Here's the drawing with two shaded views (mm, measured from the low corner). I have some questions. A direction names the side the tool comes from. Coordinates: 2 decimals unless noted, no trailing zeros. Use one line per item in the form item = value.
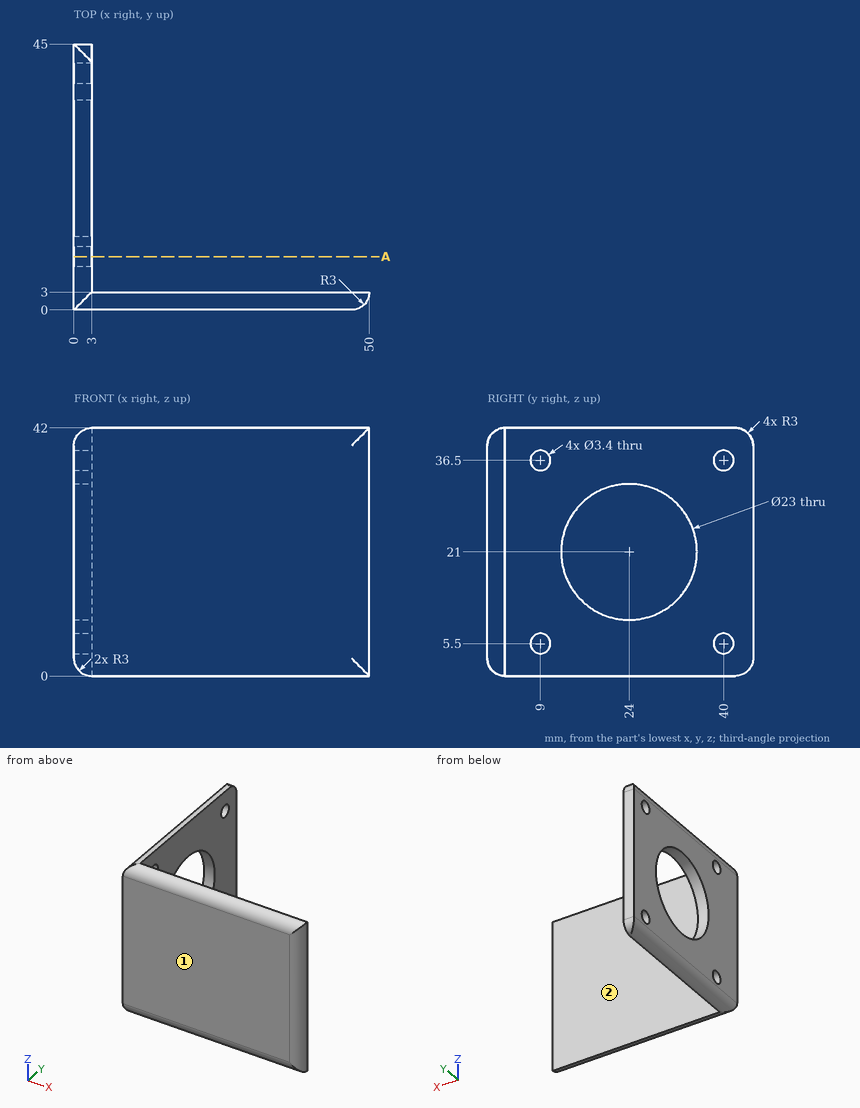
Q1. For the marked faces 1 and 2, which set-ups out of +Z, -Z, +X, -X, +Y, -Y let a thin tool reach every point of the face, with its end or its side?
Return value:
face_1 = +Z, -Z, +X, -X, -Y
face_2 = +Z, -Z, +X, +Y
Q2. Will these pins go through, and if not, where does the flat tip stop? pin 1 (3 mm diameter, centred on y = 9, z = 36.5, fed in from +X); pin 2 (1.5 mm diameter, centred on x = 39, z = 10, fed in from +Y); pin 3 (12.5 mm diameter, centred on y = 25.5, z = 26.5, fed in from +X).
Return value:
pin_1 = through
pin_2 = 3
pin_3 = 3
Q3. If I drill on line 1 (Z direction, x = 1, y = 9); line 2 (Z direction, x = 1.1, y = 40); line 3 (X direction, y = 13.5, z = 9), over which ranges is the centre line in solid material (lowest first)? Write a range as from..to.
Return value:
line_1 = 0.76..3.8, 7.2..34.8, 38.2..41.24
line_2 = 0.68..3.8, 7.2..34.8, 38.2..41.32
line_3 = 0..3
Q4. Suppose I cut it at A-A (y = 9). Give the number of separate pieces and of enclosed holes in the cut face, then the cut area to 3 significant figures.
Return value:
separate_pieces = 3
enclosed_holes = 0
area = 102 mm2
